Part model, mm, in its own coordinate system. Coordinates: 2 decimals unless noted, no trailing zeros. Loops run counter-clockwise (first coordinate to the right, second up) from the corner with the lowest first, then second, coordinate; pieces in that order, holes last. Notation, with made-up numbers: (83.25, -36.5) -> (99.25, -36.5) arc R21 ccw to (99.25, -17.5) -> close; hole circle Ø8 at (7.25, -24). An arc over 180 degrees is marked (long way). One line per item, written item: value. Start each with the question number.
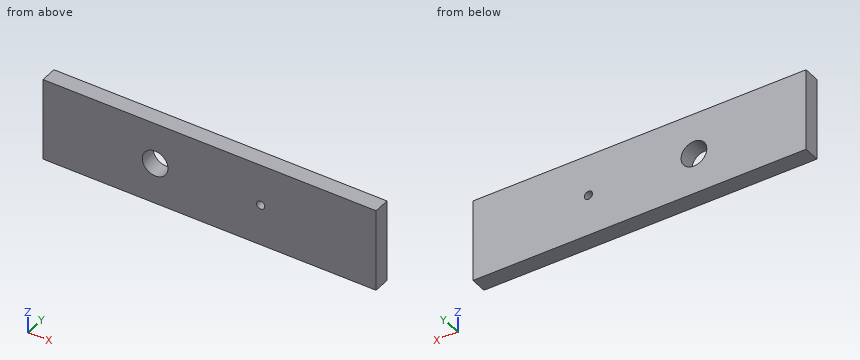
Autodesk Inventor part; units mm, degrees
ref_plane "YZ Plane" through (0, 0, 0) normal (1, 0, 0) x (0, 1, 0)
ref_plane "XZ Plane" through (0, 0, 0) normal (0, 1, 0) x (-1, 0, 0)
ref_plane "XY Plane" through (0, 0, 0) normal (0, 0, 1) x (1, 0, 0)
sketch "Sketch1" plane through (0, 0, 0) normal (0, 1, 0) x (-1, 0, 0)
  line L0 (0, 0) -> (202, 0)
  line L1 (202, 0) -> (202, 50)
  line L2 (202, 50) -> (0, 50)
  line L3 (0, 50) -> (0, 0)
  circle A0 centre (70, 25) radius 2.5
  circle A1 centre (134, 25) radius 7.8
extrude "Extrusion1" add sketch "Sketch1" along normal blind 10
properties part number "column" material "Wood (Oak)"
1) Probe line 1 (Z direction, x = -70, y = 7.25); line 2 (Z direction, x = -134, y = 3.5); line 3 (X direction, y = 5, z = 23). List the from-to ranges inside material, lowest first. Write a range as from..to.
2) Slice it at B-B (z = 25). Give the cut face in (x, y), then the cut area to 3 significant figures.
3) Pin check, flat tip, straight feed: pin 1 Ø9.5 at (x, z) = (-134, 25) entering from +Y. Stop position of the tip, or through.
4) Slice it at C-C (y = 8.5). Give the cut face in (x, z), then the cut area to 3 significant figures.
5) Slice it at A-A (x = -134). Give the cut face in (y, z).
6) Slice it at D-D (x = -70). Give the cut face in (y, z).
Check sheet entries:
1. line 1: z = 0..22.5, 27.5..50
1. line 2: z = 0..17.2, 32.8..50
1. line 3: x = -202..-141.54, -126.46..-71.5, -68.5..0
2. outline: (-202, 0) -> (-141.8, 0) -> (-141.8, 10) -> (-202, 10) -> close; (-126.2, 0) -> (-72.5, 0) -> (-72.5, 10) -> (-126.2, 10) -> close; (-67.5, 0) -> (0, 0) -> (0, 10) -> (-67.5, 10) -> close
2. area: 1,810 mm^2
3. pin 1: passes through
4. outline: (-202, 0) -> (0, 0) -> (0, 50) -> (-202, 50) -> close; hole circle Ø15.6 at (-134, 25); hole circle Ø5 at (-70, 25)
4. area: 9,890 mm^2
5. outline: (0, 0) -> (10, 0) -> (10, 17.2) -> (0, 17.2) -> close; (0, 32.8) -> (10, 32.8) -> (10, 50) -> (0, 50) -> close
6. outline: (0, 0) -> (10, 0) -> (10, 22.5) -> (0, 22.5) -> close; (0, 27.5) -> (10, 27.5) -> (10, 50) -> (0, 50) -> close
